```python
from build123d import *

# Parameters (mm, degrees)
SKETCH_R     = 7
PAD_DEPTH    = 2
PAD001_DEPTH = 11
SKETCH002_W  = 3.4
SKETCH002_H  = 3.4
POCKET_DEPTH = 8.5
FILLET_R     = 0.2
FILLET001_R  = 0.2
CHAMFER_SIZE = 1.6
FILLET002_R  = 0.5


with BuildPart() as part:
    # Sketch → Pad (new body)
    with BuildSketch(Plane.XY):
        Circle(SKETCH_R)
    extrude(amount=PAD_DEPTH)

    # Sketch001 (on Face3 of Pad) → Pad001 (join)
    with BuildSketch(Plane.XY.offset(2)):
        with BuildLine():
            ThreePointArc((-1.27, 2.495416), (-1.979899, 1.979899), (-2.495416, 1.27))
            Line((-2.495416, 1.27), (-3.895416, 1.27))
            Line((-3.895416, 1.27), (-3.895416, -1.27))
            Line((-3.895416, -1.27), (-2.495416, -1.27))
            ThreePointArc((-2.495416, -1.27), (-1.979899, -1.979899), (-1.27, -2.495416))
            Line((-1.27, -2.495416), (-1.27, -3.895416))
            Line((-1.27, -3.895416), (1.27, -3.895416))
            Line((1.27, -3.895416), (1.27, -2.495416))
            ThreePointArc((1.27, -2.495416), (1.979899, -1.979899), (2.495416, -1.27))
            Line((3.895416, -1.27), (2.495416, -1.27))
            Line((3.895416, 1.27), (3.895416, -1.27))
            Line((2.495416, 1.27), (3.895416, 1.27))
            ThreePointArc((2.495416, 1.27), (1.979899, 1.979899), (1.27, 2.495416))
            Line((1.27, 3.895416), (1.27, 2.495416))
            Line((-1.27, 3.895416), (1.27, 3.895416))
            Line((-1.27, 2.495416), (-1.27, 3.895416))
        make_face()
    extrude(amount=PAD001_DEPTH)

    # Sketch002 (on Face2 of Pad001) → Pocket (cut)
    with BuildSketch(Plane(origin=(0, 0, 0), x_dir=(1, 0, 0), z_dir=(0, 0, -1))):
        Rectangle(SKETCH002_W, SKETCH002_H)
    extrude(amount=-POCKET_DEPTH, mode=Mode.SUBTRACT)

    # Fillet
    fillet_edges = [part.edges().sort_by_distance(p)[0] for p in [
        (-3.895416, -1.27, 7.5),
        (-1.27, -3.895416, 7.5),
        (1.27, -3.895416, 7.5),
        (3.895416, -1.27, 7.5),
        (3.895416, 1.27, 7.5),
        (1.27, 3.895416, 7.5),
        (-1.27, 3.895416, 7.5),
        (-3.895416, 1.27, 7.5),
    ]]
    fillet(fillet_edges, radius=FILLET_R)

    # Fillet001
    fillet001_edges = [part.edges().sort_by_distance(p)[0] for p in [
        (1.27, 3.095416, 2),
        (1.211421, 3.836837, 2),
        (1.979899, 1.979899, 2),
        (0, 3.895416, 2),
        (3.095416, 1.27, 2),
        (-1.211421, 3.836837, 2),
        (3.836837, 1.211421, 2),
        (-1.27, 3.095416, 2),
        (3.895416, 0, 2),
        (-1.979899, 1.979899, 2),
        (3.836837, -1.211421, 2),
        (-3.095416, 1.27, 2),
        (3.095416, -1.27, 2),
        (-3.836837, 1.211421, 2),
        (1.979899, -1.979899, 2),
        (-3.895416, 0, 2),
        (1.27, -3.095416, 2),
        (-3.836837, -1.211421, 2),
        (1.211421, -3.836837, 2),
        (-3.095416, -1.27, 2),
        (0, -3.895416, 2),
        (-1.979899, -1.979899, 2),
        (-1.211421, -3.836837, 2),
        (-1.27, -3.095416, 2),
        (-7, 0, 2),
    ]]
    fillet(fillet001_edges, radius=FILLET001_R)

    # Chamfer
    chamfer_edges = [part.edges().sort_by_distance(p)[0] for p in [
        (-1.7, 0, 8.5),
        (0, -1.7, 8.5),
        (1.7, 0, 8.5),
        (0, 1.7, 8.5),
    ]]
    chamfer(chamfer_edges, length=CHAMFER_SIZE)

    # Fillet002
    fillet002_edges = [part.edges().sort_by_distance(p)[0] for p in [
        (-1.7, 1.7, 3.45),
        (-1.7, -1.7, 3.45),
        (1.7, -1.7, 3.45),
        (1.7, 1.7, 3.45),
    ]]
    fillet(fillet002_edges, radius=FILLET002_R)


solid = part.part
```
Verification items for the finished model (mm, model axes). A direction names the side the tool comes from. Coordinates: 2 decimals unless noted, no trailing zeros. Write each loop counter-clockwise with the first axis right and the second up, starting at its lowest first coordinate (ties: lowest second). Pieces come first, ordered by that corner, then holes. Notation, with made-up numbers: M -2,4 L 27,4 A15 cw 27,18 Z; hole C 25,73.5 d5. An arc over 180 degrees is marked long. Answer as a JSON object with one key per item and string values. Group by question number.
(1) Gauge pin test, flat ends, axial feed: pin 1 (5 mm diameter, centred on x = 0, z = 11.5, fed in from +Y); pin 2 (0.6 mm diameter, centred on x = -3, z = 9, fed in from -Y); pin 3 (1.7 mm diameter, centred on y = 0, z = 6.5, fed in from +X). Record the tip position at first contact, or that the pin passes through.
(2) Release check for a two-part mould opening along X. For faces 1 (the face through (0, 1.1, 7.5)), 2 (the face through (-1.99, -1.97, 7.52)), 3 (the face through (1.27, 3, 8)) record: +X half, -X half, draft (parallel to the pull), parting line (faces both ways), or undercut.
(3) Material ranges on line 1 (Y direction, x = -1, z = 3.75); line 2 (Y direction, x = 0.25, z = 1), recorded low to high.
(4) Tool access check on faces 4 (the face through (-1.27, -3, 8)), 5 (the face through (-1.1, 0, 7.5)), 6 (the face through (1.27, -3, 8)). Record the directions out of +Z, -Z, +X, -X, +Y, -Y that give a thin tool (end or side, any length) a straight path to the whole face; none if there is none.
(5) Cross-section at B-B, the plane z = 12.25. Record the cut outline in (x, y), and give its area (3 significant figures).
Reply:
{
 "1": {"pin 1": "y = 3.9", "pin 2": "y = -1.27", "pin 3": "x = 3.9"},
 "2": {"face 1": "undercut", "face 2": "-X half", "face 3": "+X half"},
 "3": {"line 1": "-3.9 to -1.7, 1.7 to 3.9", "line 2": "-7 to -1.7, 1.7 to 7"},
 "4": {"face 4": "+Z, -X, -Y", "face 5": "-Z", "face 6": "+Z, +X, -Y"},
 "5": {"outline": "M -3.9,-1.07 A0.2 ccw -3.7,-1.27 L -2.5,-1.27 A2.8 ccw -1.27,-2.5 L -1.27,-3.7 A0.2 ccw -1.07,-3.9 L 1.07,-3.9 A0.2 ccw 1.27,-3.7 L 1.27,-2.5 A2.8 ccw 2.5,-1.27 L 3.7,-1.27 A0.2 ccw 3.9,-1.07 L 3.9,1.07 A0.2 ccw 3.7,1.27 L 2.5,1.27 A2.8 ccw 1.27,2.5 L 1.27,3.7 A0.2 ccw 1.07,3.9 L -1.07,3.9 A0.2 ccw -1.27,3.7 L -1.27,2.5 A2.8 ccw -2.5,1.27 L -3.7,1.27 A0.2 ccw -3.9,1.07 Z", "area": "36.7 mm²"}
}
